Build history of the part. All positions in model axes, mm. Give positions to 0.01 mm unless a question says otherwise; leave off trailing zeros. Order: outer loops, then holes, each group sorted by start corner. A loop starts at its lowest first (then second) coordinate and runs counter-clockwise, first axis right, second up. Notation, with made-up numbers: (-13, 74) - (-2, 74) arc R28 ccw to (-2, 108) - close; hole circle Ø9 at (48, 82). An arc over 180 degrees is marked (long way). Answer in a Markdown table with one row per item.
```python
from build123d import *

# Parameters (mm, degrees)
F0_W     = 80
F0_H     = 130
F0_R     = 3.5
F0_R_2   = 4.5
F1_DEPTH = 6
F2_R     = 20


with BuildPart() as f1:
    # F0 (on Front) → F1 (new body)
    with BuildSketch(Plane.XZ):
        with Locations((5.364077, 0)):
            Rectangle(F0_W, F0_H)
        with Locations((-19.635923, -55)):
            Circle(F0_R, mode=Mode.SUBTRACT)
        with Locations((30.364077, -55)):
            Circle(F0_R, mode=Mode.SUBTRACT)
        with Locations((-21.635923, 2)):
            Circle(F0_R_2, mode=Mode.SUBTRACT)
        with Locations((-4.635923, 54)):
            Circle(F0_R_2, mode=Mode.SUBTRACT)
        with Locations((35.364077, 18)):
            Circle(F0_R_2, mode=Mode.SUBTRACT)
    extrude(amount=F1_DEPTH)

    # F2
    f2_edges = [f1.edges().sort_by_distance(p)[0] for p in [
        (45.364077, -3, 65),
        (-34.635923, -3, 65),
        (-34.635923, -3, -65),
        (45.364077, -3, -65),
    ]]
    fillet(f2_edges, radius=F2_R)


solid = f1.part
```
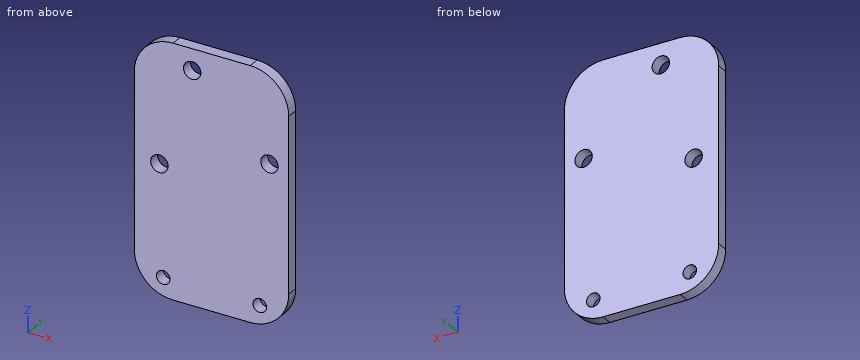
1. Drop flat-ended pins along their axis: P1, Ø1.5, axis at y = -4.5, z = -52, coming from the -X side; P2, Ø1.5, axis at x = 34.5, y = -5.5, coming from the -Z side; P3, Ø6, axis at x = -15.5, z = 14, coming from the +Y side. Give the stop position or say it passes through.
Check result:
| item | result |
|---|---|
| P1 | stops at x = -33.63 |
| P2 | stops at z = -63.16 |
| P3 | stops at y = 0 |
2. Cut at C-C on x = 32.5. Write the cut outline in (y, z), and give its area (3 significant figures).
Check result:
| item | result |
|---|---|
| outline | (-6, -63.68) - (0, -63.68) - (0, -57.77) - (-6, -57.77) - close; (-6, -52.23) - (0, -52.23) - (0, 14.53) - (-6, 14.53) - close; (-6, 21.47) - (0, 21.47) - (0, 63.68) - (-6, 63.68) - close |
| area | 689 mm² |
3. Cut at B-B on y = -1.6. Write the cut outline in (x, z).
Check result:
| item | result |
|---|---|
| outline | (-34.64, -45) arc R20 ccw to (-14.64, -65) - (25.36, -65) arc R20 ccw to (45.36, -45) - (45.36, 45) arc R20 ccw to (25.36, 65) - (-14.64, 65) arc R20 ccw to (-34.64, 45) - close; hole circle Ø9 at (-21.64, 2); hole circle Ø7 at (-19.64, -55); hole circle Ø9 at (-4.64, 54); hole circle Ø7 at (30.36, -55); hole circle Ø9 at (35.36, 18) |
4. Probe line 1 (Z direction, x = -20.5, y = -5.1); line 2 (Z direction, x = -17, y = -0.25); line 3 (Z direction, x = -2, y = -0.25). List the from-to ranges inside material, lowest first.
Check result:
| item | result |
|---|---|
| line 1 | z = -64.12 to -58.39, -51.61 to -2.35, 6.35 to 64.12 |
| line 2 | z = -64.86 to -57.3, -52.7 to 64.86 |
| line 3 | z = -65 to 50.35, 57.65 to 65 |
5. Cut at A-A on z = 18. Write the cut outline in (x, y), and give its area (3 significant figures).
Check result:
| item | result |
|---|---|
| outline | (-34.64, -6) - (30.86, -6) - (30.86, 0) - (-34.64, 0) - close; (39.86, -6) - (45.36, -6) - (45.36, 0) - (39.86, 0) - close |
| area | 426 mm² |
6. Cut at D-D on z = -55. Write the cut outline in (x, y), and give its area (3 significant figures).
Check result:
| item | result |
|---|---|
| outline | (-31.96, -6) - (-23.14, -6) - (-23.14, 0) - (-31.96, 0) - close; (-16.14, -6) - (26.86, -6) - (26.86, 0) - (-16.14, 0) - close; (33.86, -6) - (42.68, -6) - (42.68, 0) - (33.86, 0) - close |
| area | 364 mm² |
